For this review, use the dimensioned drawing (mm, ordinates from the lowest corner) and the shaded views. Coordinates: 2 decimals unless noted, no trailing zeros. Write each loop counter-clockwise with the first axis right and the second up, starting at its lowest first coordinate (ties: lowest second). Pieces come first, ordered by that corner, then holes. Notation, with made-up numbers: (50.25, 88.5) - (103.25, 88.5) arc R20 ccw to (103.25, 121.5) - close; hole circle Ø9 at (-36, 27). An arc over 180 degrees is marked (long way). Put each result on its own line as item: value.
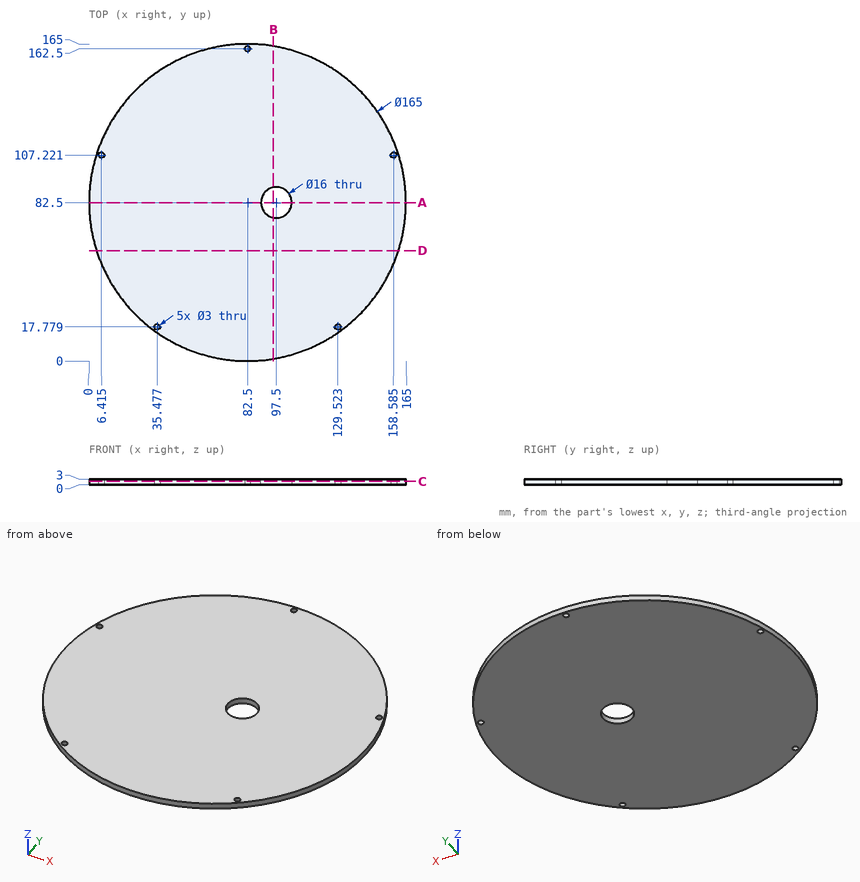
1. Consider section B-B on x = 96. State the section outline as (y, z) points.
Determined:
outline: (1.11, 0) - (74.64, 0) - (74.64, 3) - (1.11, 3) - close; (90.36, 0) - (163.89, 0) - (163.89, 3) - (90.36, 3) - close
2. Consider section D-D on y = 57.5. State the section outline as (x, z) points.
Determined:
outline: (3.88, 0) - (161.12, 0) - (161.12, 3) - (3.88, 3) - close
3. To check wall thickness, follow probe 1 along Y at (x, z) = (82.5, 2.35); probe 2 along X at (y, z) = (108.5, 0.85) (1 decimal); probe 3 along Y at (x, z) = (97.5, 1.95) (1 decimal). State the ranges of each line that lie inside material, in increasing order.
Determined:
probe 1: y = 0 to 161, 164 to 165
probe 2: x = 4.2 to 5.6, 7.2 to 157.8, 159.4 to 160.8
probe 3: y = 1.4 to 74.5, 90.5 to 163.6
4. Consider section C-C on z = 1.7. State the section outline as (x, y) points (1 decimal), plus the area to 3 significant figures.
Determined:
outline: circle Ø165 at (82.5, 82.5); hole circle Ø3 at (6.4, 107.2); hole circle Ø3 at (35.5, 17.8); hole circle Ø3 at (82.5, 162.5); hole circle Ø16 at (97.5, 82.5); hole circle Ø3 at (129.5, 17.8); hole circle Ø3 at (158.6, 107.2)
area: 21,100 mm^2
5. Consider section A-A on y = 82.5. State the section outline as (x, z) points.
Determined:
outline: (0, 0) - (89.5, 0) - (89.5, 3) - (0, 3) - close; (105.5, 0) - (165, 0) - (165, 3) - (105.5, 3) - close
6. For pin 1 Ø2.5 at (x, y) = (35.48, 17.78) entering from +Z; pin 2 Ø1.5 at (x, z) = (147, 1) entering from +Y (1 decimal); pin 3 Ø1 at (y, z) = (32, 0.5) entering from +X, all flat-tipped, find the tip position at first contact; note any pin that passes through.
Determined:
pin 1: passes through
pin 2: stops at y = 134.9
pin 3: stops at x = 148.12
